from build123d import *

# Parameters (mm, degrees)
CROQUIS1_R              = 35
SALIENTE_EXTRUIR1_DEPTH = 37
CHAFL_N1_SIZE           = 5
CROQUIS2_R              = 25
SALIENTE_EXTRUIR2_DEPTH = 16
CROQUIS3_R              = 28.1
SALIENTE_EXTRUIR3_DEPTH = 120
SALIENTE_EXTRUIR4_START = 30
CROQUIS4_R              = 25
SALIENTE_EXTRUIR4_DEPTH = 30
SALIENTE_EXTRUIR5_START = 120
CROQUIS5_R              = 28.1
SALIENTE_EXTRUIR5_DEPTH = 120
CORTAR_EXTRUIR1_START   = -17
CROQUIS6_R              = 28.1
CROQUIS6_R_2            = 25
CORTAR_EXTRUIR1_DEPTH   = 17
CROQUIS8_R              = 28.1
CROQUIS8_R_2            = 25
CORTAR_EXTRUIR2_DEPTH   = 17


with BuildPart() as part:
    # Croquis1 → Saliente-Extruir1 (new, symmetric)
    with BuildSketch(Plane(origin=(0, 0, 0), x_dir=(0, 0, -1), z_dir=(1, 0, 0))):
        Circle(CROQUIS1_R)
    extrude(amount=SALIENTE_EXTRUIR1_DEPTH, both=True)

    # Chaflán1
    chafl_n1_edges = [part.edges().sort_by_distance(p)[0] for p in [
        (-37, 0, 35),
        (37, 0, 35),
    ]]
    chamfer(chafl_n1_edges, length=CHAFL_N1_SIZE)

    # Croquis2 → Saliente-Extruir2 (add)
    with BuildSketch(Plane.ZY.offset(37)):
        Circle(CROQUIS2_R)
    extrude(amount=SALIENTE_EXTRUIR2_DEPTH)

    # Croquis3 → Saliente-Extruir3 (add)
    with BuildSketch(Plane.ZY.offset(53)):
        Circle(CROQUIS3_R)
    extrude(amount=SALIENTE_EXTRUIR3_DEPTH)

    # Croquis4 → Saliente-Extruir4 (add)
    with BuildSketch(Plane(origin=(37, 0, 0), x_dir=(0, 0, -1), z_dir=(1, 0, 0)).offset(SALIENTE_EXTRUIR4_START)):
        with Locations(Location((0, 0, 0), (0, 0, 180))):
            Circle(CROQUIS4_R)
    extrude(amount=-SALIENTE_EXTRUIR4_DEPTH)

    # Croquis5 → Saliente-Extruir5 (add)
    with BuildSketch(Plane(origin=(67, 0, 0), x_dir=(0, 0, -1), z_dir=(1, 0, 0)).offset(SALIENTE_EXTRUIR5_START)):
        with Locations(Location((0, 0, 0), (0, 0, 180))):
            Circle(CROQUIS5_R)
    extrude(amount=-SALIENTE_EXTRUIR5_DEPTH)

    # Croquis6 → Cortar-Extruir1 (cut)
    with BuildSketch(Plane.ZY.offset(173).offset(CORTAR_EXTRUIR1_START)):
        Circle(CROQUIS6_R)
        Circle(CROQUIS6_R_2, mode=Mode.SUBTRACT)
    extrude(amount=CORTAR_EXTRUIR1_DEPTH, mode=Mode.SUBTRACT)

    # Croquis8 → Cortar-Extruir2 (cut)
    with BuildSketch(Plane(origin=(187, 0, 0), x_dir=(0, 0, -1), z_dir=(1, 0, 0))):
        with Locations(Location((0, 0, 0), (0, 0, 180))):
            Circle(CROQUIS8_R)
        with Locations(Location((0, 0, 0), (0, 0, 180))):
            Circle(CROQUIS8_R_2, mode=Mode.SUBTRACT)
    extrude(amount=-CORTAR_EXTRUIR2_DEPTH, mode=Mode.SUBTRACT)


solid = part.part
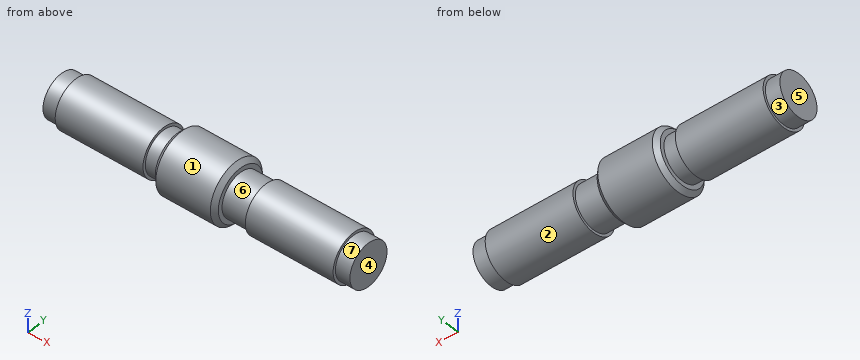
CAD build for the part. Positions are in the model's coordinates, mm. Face numbers are marked on the shaded views. A direction names the side the tool comes from. Coordinates: 2 decimals unless noted, no trailing zeros. Write each loop counter-clockwise with the first axis right and the second up, starting at its lowest first coordinate (ties: lowest second). Pieces come first, ordered by that corner, then holes. Notation, with made-up numbers: (21.25, 23) - (46.25, 23) arc R33 cw to (46.25, 60) - close; hole circle Ø6 at (13, 29.25). An arc over 180 degrees is marked (long way). Use a Markdown table: item, result. Add a question column.
Item 1: Band-saw the part on C-C, the plane x = 15.5. Give the cut face in (y, z).
Item 2: Flat gauge pins, fed straight in: pin 1 (1 mm diameter, centred on x = -67.5, y = -16.5, fed in from -Z); pin 2 (10 mm diameter, centred on y = 4.5, z = -27, fed in from -X); pin 3 (8 mm diameter, centred on x = 105.5, y = -19, fed in from -Z); pin 4 (1 mm diameter, centred on x = 82.5, y = 16, fed in from -Z). Where does each tip first touch, or does it go through?
Item 3: Band-saw the part on D-D, the plane x = 60. Give the cut face in (y, z).
Item 4: Drill centre lines: L1, parallel to X at y = -17.5, z = -20.5; L2, parallel to X at y = 15, z = 24.5; L3, parallel to Y at x = 115.5, z = 1. Where is each one in solid material? Low to high. Write a range as from..to.
Item 5: Mould opens along X. For the marked faces 4, 5, 6 and 7 say: pulls with the +X half, pulls with the -X half, needs draft (parallel to the pull), parting line crosses it, or undercut.
Item 6: 3-axis set-ups, long thin cutter, end or side, ignore diameter. For the marked faces 1, 2 and 3: which of +Z, -Z, +X, -X, +Y, -Y reach the whole face in a straight line?
Numbers:
| question | item | result |
|---|---|---|
| 1 | outline | circle Ø70 at (0, 0) |
| 2 | pin 1 | z = -23.1 |
| 2 | pin 2 | x = -173 |
| 2 | pin 3 | z = -23.76 |
| 2 | pin 4 | z = -23.44 |
| 3 | outline | circle Ø50 at (0, 0) |
| 4 | L1 | -156..-53, -37..37, 67..170 |
| 4 | L2 | -37..37 |
| 4 | L3 | -28.08..28.08 |
| 5 | face 4 | pulls with the +X half |
| 5 | face 5 | pulls with the -X half |
| 5 | face 6 | undercut |
| 5 | face 7 | needs draft |
| 6 | face 1 | +X, -X |
| 6 | face 2 | +X |
| 6 | face 3 | -X |
